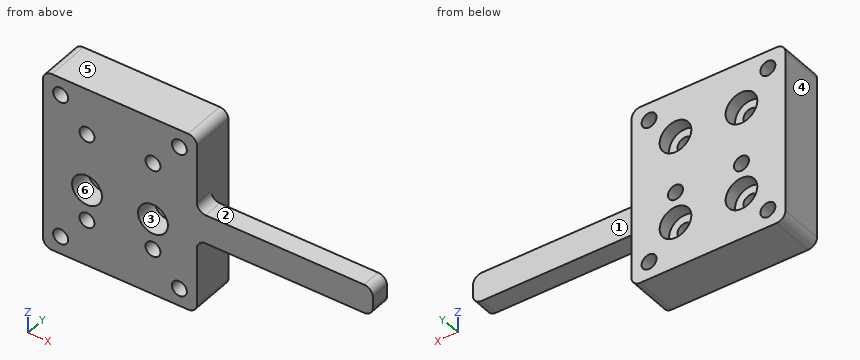
from build123d import *

# Parameters (mm, degrees)
SKETCH_1_W          = 35
SKETCH_1_H          = 41
SKETCH_1_R          = 1.7
EXTRUDE_1_DEPTH     = 10
SKETCH_2_R          = 3.6
CUT_EXTRUDE_1_DEPTH = 3
SKETCH_3_R          = 3.4
CUT_EXTRUDE_2_DEPTH = 5
SKETCH_4_R          = 1.7
CUT_EXTRUDE_3_DEPTH = 11
FILLET_1_R          = 2
SKETCH_5_W          = 6.562454648
SKETCH_5_H          = 4.478703739
EXTRUDE_2_DEPTH     = 40
FILLET_2_R          = 2


with BuildPart() as part:
    # 草图1 → 凸台-拉伸1 (new body)
    with BuildSketch(Plane(origin=(0, 0, 0), x_dir=(1, 0, 0), z_dir=(0, 1, 0))):
        with Locations((-19.214285714, 4.857142857)):
            Rectangle(SKETCH_1_W, SKETCH_1_H)
        with Locations((-26.714285714, 14.857142857)):
            Circle(SKETCH_1_R, mode=Mode.SUBTRACT)
        with Locations((-11.714285714, 14.857142857)):
            Circle(SKETCH_1_R, mode=Mode.SUBTRACT)
        with Locations((-11.714285714, -5.142857143)):
            Circle(SKETCH_1_R, mode=Mode.SUBTRACT)
        with Locations((-26.714285714, -5.142857143)):
            Circle(SKETCH_1_R, mode=Mode.SUBTRACT)
        with Locations((-11.714285714, 7.857142857)):
            Circle(SKETCH_1_R, mode=Mode.SUBTRACT)
        with Locations((-26.714285714, 7.857142857)):
            Circle(SKETCH_1_R, mode=Mode.SUBTRACT)
    extrude(amount=EXTRUDE_1_DEPTH)

    # 草图2 → 切除-拉伸1 (cut)
    with BuildSketch(Plane(origin=(0, 10, 0), x_dir=(1, 0, 0), z_dir=(0, 1, 0))):
        with Locations((-26.714285714, -5.142857143)):
            Circle(SKETCH_2_R)
        with Locations((-11.714285714, -5.142857143)):
            Circle(SKETCH_2_R)
        with Locations((-11.714285714, 14.857142857)):
            Circle(SKETCH_2_R)
        with Locations((-26.714285714, 14.857142857)):
            Circle(SKETCH_2_R)
    extrude(amount=-CUT_EXTRUDE_1_DEPTH, mode=Mode.SUBTRACT)

    # 草图3 → 切除-拉伸2 (cut)
    with BuildSketch(Plane.XZ):
        with Locations((-11.714285714, -7.857142857)):
            Circle(SKETCH_3_R)
        with Locations((-26.714285714, -7.857142857)):
            Circle(SKETCH_3_R)
    extrude(amount=-CUT_EXTRUDE_2_DEPTH, mode=Mode.SUBTRACT)

    # 草图4 → 切除-拉伸3 (cut, through all)
    with BuildSketch(Plane(origin=(0, 10, 0), x_dir=(1, 0, 0), z_dir=(0, 1, 0))):
        with Locations((-32.714285714, 21.357142857)):
            Circle(SKETCH_4_R)
        with Locations((-5.714285714, 21.357142857)):
            Circle(SKETCH_4_R)
        with Locations((-5.714285714, -11.642857143)):
            Circle(SKETCH_4_R)
        with Locations((-32.714285714, -11.642857143)):
            Circle(SKETCH_4_R)
    extrude(amount=-CUT_EXTRUDE_3_DEPTH, mode=Mode.SUBTRACT)

    # 圆角1
    fillet_1_edges = [part.edges().sort_by_distance(p)[0] for p in [
        (-36.714285714, 5, -25.357142857),
        (-1.714285714, 5, -25.357142857),
        (-1.714285714, 5, 15.642857143),
        (-36.714285714, 5, 15.642857143),
    ]]
    fillet(fillet_1_edges, radius=FILLET_1_R)

    # 草图5 → 凸台-拉伸2 (add)
    with BuildSketch(Plane(origin=(-1.714285714, 0, 0), x_dir=(0, 0, -1), z_dir=(1, 0, 0))):
        with Locations((4.857142857, 2.23935187)):
            Rectangle(SKETCH_5_W, SKETCH_5_H)
    extrude(amount=EXTRUDE_2_DEPTH)

    # 圆角2
    fillet_2_edges = [part.edges().sort_by_distance(p)[0] for p in [
        (-1.714285714, 2.239351869, -8.138370181),
        (-1.714285714, 2.239351869, -1.575915533),
        (38.285714286, 2.239351869, -8.138370181),
        (38.285714286, 2.239351869, -1.575915533),
    ]]
    fillet(fillet_2_edges, radius=FILLET_2_R)


solid = part.part
Verification items for the finished model (mm, model axes). Face numbers are marked on the shaded views. A direction names the side the tool comes from. Give positions to 0.01 mm unless a question says otherwise; leave off trailing zeros. Loops run counter-clockwise (first coordinate to the right, second up) from the corner with the lowest first, then second, coordinate; pieces in that order, holes last. Notation, with made-up numbers: (52, -5.75) - (105, -5.75) arc R9 cw to (105, 11.25) - close; hole circle Ø3 at (-39.75, 55). An arc over 180 degrees is marked (long way). Write item = value, one per line. Start each with the question number.
Q1. Cross-section at A-A, the plane x = -27. Enter the section's corners in (y, z).
Q2. Thickness scan on line 1 (X direction, y = 4.25, z = -21.5); line 2 (X direction, y = 5.5, z = 5); line 3 (Z direction, x = -11, y = 7.5). Record the ranges inside material, lowest first.
Q3. Cross-section at B-B, the plane y = 8.75. State how many separate pieces and enclosed holes the cut face has, and give its area (3 significant figures).
Q4. Cross-section at C-C, the plane x = 24. Enter the section's corners in (y, z), and give its area (3 significant figures).
Q5. Tool access check on the marked faces 1, 2 and 3. Record the directions out of +Z, -Z, +X, -X, +Y, -Y that give a thin tool (end or side, any length) a straight path to the whole face; none if there is none.
Q6. Mould release check, pull along X, two halves, no side actions. Record for the marked faces 4, 5 and 6: released by +X, released by -X, zero draft, split by the parting line, or undercut.
Q7. Depth check by flat-ended pin: P1, Ø2, axis at x = -11.71, z = 5.14, coming from the +Y side; P2, Ø1.3, axis at x = 18.5, y = 1.5, coming from the +Z side; P3, Ø2, axis at x = 12.5, y = 2.5, coming from the -Z side; P4, Ø3.5, axis at x = -11, z = -13.5, coming from the +Y side. Enter the tip coordinate at first touch or a pass-through.
Q8. Cross-section at D-D, the plane z = -0.5. Enter the section's corners in (x, y), and give its area (3 significant figures).
Answer key:
q1.outline = (0, -25.36) - (10, -25.36) - (10, -18.45) - (7, -18.45) - (7, -16.53) - (0, -16.53) - close; (0, -13.18) - (7, -13.18) - (7, -11.27) - (10, -11.27) - (10, -9.53) - (5, -9.53) - (5, -11.25) - (0, -11.25) - close; (0, -4.47) - (5, -4.47) - (5, -6.18) - (10, -6.18) - (10, 1.55) - (7, 1.55) - (7, 3.47) - (0, 3.47) - close; (0, 6.82) - (7, 6.82) - (7, 8.73) - (10, 8.73) - (10, 15.64) - (0, 15.64) - close
q2.line_1 = -36.71 to -34.41, -31.02 to -7.41, -4.02 to -1.71
q2.line_2 = -36.71 to -28.41, -25.02 to -13.41, -10.02 to -1.71
q2.line_3 = -25.36 to -18.39, -11.33 to -9.4, -6.31 to 1.61, 8.67 to 15.64
q3.separate_pieces = 1
q3.enclosed_holes = 10
q3.area = 1,210 mm^2
q4.outline = (0, -8.14) - (4.48, -8.14) - (4.48, -1.58) - (0, -1.58) - close
q4.area = 29.4 mm^2
q5.face_1 = +Z, -Z, +X, +Y
q5.face_2 = +Z, +X, +Y, -Y
q5.face_3 = -Y
q6.face_4 = released by -X
q6.face_5 = zero draft
q6.face_6 = undercut
q7.P1 = through
q7.P2 = -1.58
q7.P3 = -8.14
q7.P4 = 7
q8.outline = (-36.71, 0) - (-1.49, 0) - (-1.49, 4.48) - (-1.71, 4.48) - (-1.71, 10) - (-36.71, 10) - close
q8.area = 351 mm^2
